Source: CAD feature listing. Evaluate the final solid. Frame: model axes, mm. Face numbers are marked on the shaded views. A direction names the side the tool comes from. Give positions to 0.01 mm unless a question says otherwise; leave off trailing zeros. Order: outer loops, then holes, each group sorted by start corner. A loop starts at its lowest first (then second) coordinate and runs counter-clockwise, first axis right, second up. Notation, with made-up numbers: (-8.75, 9) -> (43.25, 9) arc R10 cw to (43.25, 22) -> close; hole circle Ø5 at (-36.5, -20). An arc over 180 degrees is marked (long way). Answer in a Markdown table with one row per item.
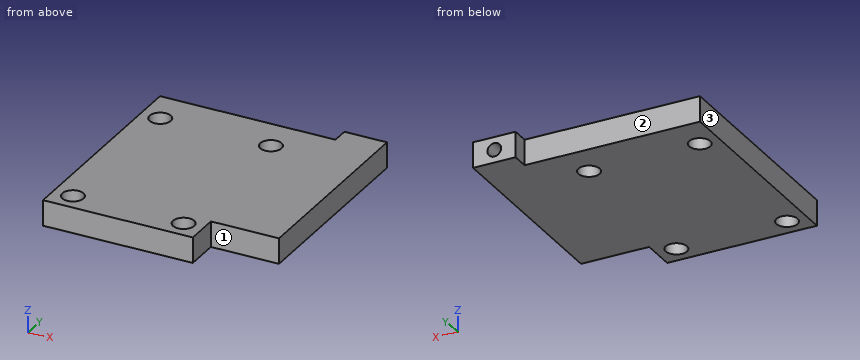
Autodesk Inventor part; units mm, degrees
ref_plane "作業平面1" through (0, 0, 0) normal (0, 0, 1) x (1, 0, 0)
ref_plane "YZ Plane" through (0, 0, 0) normal (1, 0, 0) x (0, 1, 0)
ref_plane "XZ Plane" through (0, 0, 0) normal (0, 1, 0) x (-1, 0, 0)
ref_plane "作業平面1" through (0, 0, 0) normal (0, 0, 1) x (1, 0, 0)
sketch "スケッチ1" plane through (0, 0, 0) normal (0, 0, 1) x (1, 0, 0)
  circle A0 centre (-6, -21.7) radius 1.25
  circle A1 centre (-19, -21.7) radius 1.25
  circle A2 centre (-19, -2.3) radius 1.25
  circle A3 centre (-6, -2.3) radius 1.25
  line L0 (0, -24) -> (-27.3, -24)
  line L1 (-3.7, -24) -> (-3.7, 2)
  line L2 (-3.7, 2) -> (-21.3, 2)
  line L3 (-21.3, 2) -> (-21.3, -24)
  circle A4 centre (-6, -21.7) radius 2.3 construction
  circle A5 centre (-19, -21.7) radius 2.3 construction
  line L4 (-3.7, -20) -> (4.3, -20)
  line L5 (4.3, -20) -> (4.3, 4)
  line L6 (4.3, 4) -> (-0.7, 4)
  line L7 (-0.7, 4) -> (-0.7, 2)
  line L8 (-0.7, 2) -> (-3.7, 2)
  point P0 (0, 0)
  dimension "d0" = 26
  dimension "d3" = 3
  dimension "d4" = 5
  dimension "d5" = 2
  dimension "d6" = 24
extrude "押し出し1" add sketch "スケッチ1" along normal blind 3
sketch "スケッチ2" plane through (-0.7, 4, 0) normal (0, 1, 0) x (1, 0, 0)
  line L0 (5, 0) -> (0, 0)
  line L1 (0, 0) -> (0, -3)
  line L2 (5, -3) -> (0, -3)
  line L3 (5, 0) -> (5, -3)
  circle A0 centre (2.5, -1.5) radius 0.8
  line L4 (5, -3) -> (0, 0) construction
  line L5 (5, 0) -> (0, -3) construction
  point P0 (0.7, 0)
  dimension "d7" = 1.6
extrude "押し出し2" cut sketch "スケッチ2" against normal blind 5 contours A0
properties part number "KickerMount_R"
(1) Section query C-C (z = 2.65). Return the cut outline in (x, y), plus the area to 3 significant figures.
A:
| item | result |
|---|---|
| outline | (-21.3, -24) -> (-3.7, -24) -> (-3.7, -20) -> (4.3, -20) -> (4.3, 4) -> (-0.7, 4) -> (-0.7, 2) -> (-21.3, 2) -> close; hole circle Ø2.5 at (-19, -21.7); hole circle Ø2.5 at (-19, -2.3); hole circle Ø2.5 at (-6, -21.7); hole circle Ø2.5 at (-6, -2.3) |
| area | 624 mm^2 |
(2) Section query D-D (y = 0.5). Return the cut outline in (x, z), plus the area to 3 significant figures.
A:
| item | result |
|---|---|
| outline | (-21.3, 0) -> (4.3, 0) -> (4.3, 3) -> (-21.3, 3) -> close; hole circle Ø1.6 at (1.8, 1.5) |
| area | 74.8 mm^2 |
(3) First-contact query: pin 1 Ø4 at (x, y) = (-19, -2.3) entering from -Z; pin 2 Ø0.9 at (x, z) = (-11, 1.5) entering from +Y; pin 3 Ø0.5 at (x, z) = (1.5, 1.5) entering from +Y; pin 4 Ø1.6 at (y, z) = (3.5, 1) entering from -X. Flat tips, straight axial feed; report the tip coordinate or a pass-through.
A:
| item | result |
|---|---|
| pin 1 | stops at z = 0 |
| pin 2 | stops at y = 2 |
| pin 3 | stops at y = -1 |
| pin 4 | stops at x = -0.7 |
(4) Section query A-A (x = -6). Return the cut outline in (y, z), plus the area to 3 significant figures.
A:
| item | result |
|---|---|
| outline | (-24, 0) -> (-22.95, 0) -> (-22.95, 3) -> (-24, 3) -> close; (-20.45, 0) -> (-3.55, 0) -> (-3.55, 3) -> (-20.45, 3) -> close; (-1.05, 0) -> (2, 0) -> (2, 3) -> (-1.05, 3) -> close |
| area | 63.0 mm^2 |
(5) Access query for the marked faces 1, 2 and 3. Directions: +Z, -Z, +X, -X, +Y, -Y. A direction counts if a zero-diameter tool reaches every point of the face in a straight line with its end or side. Return the directions, or none.
A:
| item | result |
|---|---|
| face 1 | +Z, -Z, +X, -Y |
| face 2 | +Z, -Z, -X, +Y |
| face 3 | +Z, -Z, -X, +Y, -Y |
(6) Section query B-B (y = -21.7). Return the cut outline in (x, z), plus the area to 3 significant figures.
A:
| item | result |
|---|---|
| outline | (-21.3, 0) -> (-20.25, 0) -> (-20.25, 3) -> (-21.3, 3) -> close; (-17.75, 0) -> (-7.25, 0) -> (-7.25, 3) -> (-17.75, 3) -> close; (-4.75, 0) -> (-3.7, 0) -> (-3.7, 3) -> (-4.75, 3) -> close |
| area | 37.8 mm^2 |
(7) Ray query, probe 1 along Y at (x, z) = (-19, 2.4); probe 2 along X at (y, z) = (-1.25, 2.45); probe 3 along Y at (x, z) = (-19.5, 0.35). Return the intervals inside material, ascending.
A:
| item | result |
|---|---|
| probe 1 | y = -24 to -22.95, -20.45 to -3.55, -1.05 to 2 |
| probe 2 | x = -21.3 to -19.68, -18.32 to -6.68, -5.32 to 4.3 |
| probe 3 | y = -24 to -22.85, -20.55 to -3.45, -1.15 to 2 |
